from build123d import *

# Parameters (mm, degrees)
SKETCH_1_W          = 120
SKETCH_1_H          = 65
EXTRUDE_1_DEPTH     = 4
SKETCH_2_R          = 1.5
CUT_EXTRUDE_1_DEPTH = 4
FILLET_1_R          = 5
SKETCH_3_R          = 1.5
CUT_EXTRUDE_2_DEPTH = 4


with BuildPart() as part:
    # 草图1 → 凸台-拉伸1 (new body)
    with BuildSketch(Plane(origin=(0, 0, 0), x_dir=(1, 0, 0), z_dir=(0, 1, 0))):
        Rectangle(SKETCH_1_W, SKETCH_1_H)
    extrude(amount=EXTRUDE_1_DEPTH)

    # 草图2 → 切除-拉伸1 (cut)
    with BuildSketch(Plane(origin=(0, 4, 0), x_dir=(1, 0, 0), z_dir=(0, 1, 0))):
        with Locations(Location((50, -27.75, 0), (0, 0, 270))):
            Circle(SKETCH_2_R)
        with Locations(Location((50, 27.75, 0), (0, 0, 270))):
            Circle(SKETCH_2_R)
        with Locations(Location((30, 27.75, 0), (0, 0, 270))):
            Circle(SKETCH_2_R)
        with Locations(Location((30, -27.75, 0), (0, 0, 270))):
            Circle(SKETCH_2_R)
    cut_extrude_1 = extrude(amount=-CUT_EXTRUDE_1_DEPTH, mode=Mode.SUBTRACT)

    # 镜向2: 切除-拉伸1 across plane
    add(cut_extrude_1.mirror(Plane(origin=(0, 0, 0), x_dir=(0, 0, 1), z_dir=(1, 0, 0))), mode=Mode.SUBTRACT)

    # 圆角1
    fillet_1_edges = [part.edges().sort_by_distance(p)[0] for p in [
        (60, 2, 32.5),
        (-60, 2, 32.5),
        (-60, 2, -32.5),
        (60, 2, -32.5),
    ]]
    fillet(fillet_1_edges, radius=FILLET_1_R)

    # 草图3 → 切除-拉伸2 (cut)
    with BuildSketch(Plane(origin=(0, 4, 0), x_dir=(1, 0, 0), z_dir=(0, 1, 0))):
        with Locations(Location((-20, 25, 0), (0, 0, 270))):
            Circle(SKETCH_3_R)
        with Locations(Location((20, 25, 0), (0, 0, 270))):
            Circle(SKETCH_3_R)
        with Locations(Location((20, -25, 0), (0, 0, 270))):
            Circle(SKETCH_3_R)
        with Locations(Location((-20, -25, 0), (0, 0, 270))):
            Circle(SKETCH_3_R)
    extrude(amount=-CUT_EXTRUDE_2_DEPTH, mode=Mode.SUBTRACT)


solid = part.part
Can you work these out from the model? Positions are in its coordinate system, mm. Give positions to 0.01 mm unless a question says otherwise; leave off trailing zeros. Write each loop counter-clockwise with the first axis right and the second up, starting at its lowest first coordinate (ties: lowest second). Pieces come first, ordered by that corner, then holes. Notation, with made-up numbers: M 72,73 L 129,73 A31 ccw 129,100 Z; hole C 67,-25 d11. An arc over 180 degrees is marked long. Answer in a Markdown table with one row per item. Add a question column.
Item 1: For pin 1 Ø1.8 at (x, z) = (-30, 27.75) entering from -Y, with a flat end and sliding along its axis, tell me the tip position at first contact or that it passes through.
Item 2: Please list where these lines run through material, in increasing order: L1, parallel to X at y = 3.2, z = 25; L2, parallel to X at y = 2.5, z = 27.75; L3, parallel to X at y = 2.25, z = -24.5.
Item 3: Imagine slicing it at A-A, the plane x = -20. Write out the boundary of the cut face in (y, z), plus the area to 3 significant figures.
Item 4: We'd pull the mould along X, two halves only. Please class faces 1 (the cylindrical face through (48.536, 2.028, 27.425)), 2 (the flat face through (60, 2, 0)), 3 (the flat face through (-1, 2, -32.5)): released by +X, released by -X, zero draft, split by the parting line, or undercut.
Item 5: Imagine slicing it at B-B, the plane z = -25. Write out the boundary of the cut face in (x, y).
Evaluation:
| question | item | result |
|---|---|---|
| 1 | pin 1 | passes through |
| 2 | L1 | x = -60 to -21.5, -18.5 to 18.5, 21.5 to 60 |
| 2 | L2 | x = -59.99 to -51.5, -48.5 to -31.5, -28.5 to 28.5, 31.5 to 48.5, 51.5 to 59.99 |
| 2 | L3 | x = -60 to -21.41, -18.59 to 18.59, 21.41 to 60 |
| 3 | outline | M 0,-32.5 L 4,-32.5 L 4,-26.5 L 0,-26.5 Z; M 0,-23.5 L 4,-23.5 L 4,23.5 L 0,23.5 Z; M 0,26.5 L 4,26.5 L 4,32.5 L 0,32.5 Z |
| 3 | area | 236 mm² |
| 4 | face 1 | undercut |
| 4 | face 2 | released by +X |
| 4 | face 3 | zero draft |
| 5 | outline | M -60,0 L -21.5,0 L -21.5,4 L -60,4 Z; M -18.5,0 L 18.5,0 L 18.5,4 L -18.5,4 Z; M 21.5,0 L 60,0 L 60,4 L 21.5,4 Z |
